Input: part model. Units: mm. Frame: model coordinates. A direction names the side the tool comes from. Coordinates: 2 decimals unless noted, no trailing zeros. Write each loop counter-clockwise with the first axis right and the second up, starting at its lowest first coordinate (ties: lowest second). Pieces come first, ordered by that corner, then holes.
1) Section query C-C (z = -2.25). Output: boundary loops of the cut face in (x, y).
2) Section query B-B (z = 7). Output: boundary loops of the cut face in (x, y).
3) Set-up query: faces 1 (the flat face through (0, 0, 0)), 2 (the cylindrical face through (21.79, 1.05, 5.9)), 3 (the cylindrical face through (-21.79, 0.6, 6.523)). Return all of +Z, -Z, +X, -X, +Y, -Y with unobstructed straight access to the full face (end or side cutting, diameter ignored); none if empty.
4) Draft query along Z for faces 4 (the flat face through (-22.5, 1, 7)), 5 (the cylindrical face through (21.79, 0.6, 6.523)), 6 (the flat face through (0, 1, -8.5)). Return one class per face: pulls with the +Z half, pulls with the -Z half, needs draft (parallel to the pull), parting line crosses it, or undercut.
5) Line query: L1, parallel to X at y = 0.95, z = -5.75; L2, parallel to Z at x = 21.5, y = 0.55. Output: solid intervals per line, ascending.
from build123d import *

# Parameters (mm, degrees)
SKETCH1_W           = 42
SKETCH1_H           = 17
BOSS_EXTRUDE1_DEPTH = 1.5
SKETCH2_R           = 0.5
BOSS_EXTRUDE2_DEPTH = 1.5
FILLET1_R           = 0.1


with BuildPart() as part:
    # Sketch1 → Boss-Extrude1 (new body)
    with BuildSketch(Plane(origin=(0, 0, 0), x_dir=(1, 0, 0), z_dir=(0, 1, 0))):
        Rectangle(SKETCH1_W, SKETCH1_H)
    extrude(amount=BOSS_EXTRUDE1_DEPTH)

    # Sketch2 → Boss-Extrude2 (add)
    with BuildSketch(Plane.ZY.offset(21)):
        with Locations(Location((5.5, 0.75, 0), (0, 0, 180))):
            Circle(SKETCH2_R)
        with Locations(Location((7, 0.75, 0), (0, 0, 180))):
            Circle(SKETCH2_R)
    boss_extrude2 = extrude(amount=BOSS_EXTRUDE2_DEPTH)

    # Mirror1: Boss-Extrude2 across plane
    add(boss_extrude2.mirror(Plane(origin=(0, 0, 0), x_dir=(0, 0, 1), z_dir=(1, 0, 0))))

    # Fillet1
    fillet1_edges = [part.edges().sort_by_distance(p)[0] for p in [
        (21, 1.5, 0),
        (-21, 0.75, 7.5),
        (-21, 0.75, 6),
        (0, 1.5, -8.5),
        (21, 0.75, 6),
        (21, 0.75, 7.5),
        (-21, 1.5, 0),
        (0, 0, -8.5),
        (21, 0, 0),
        (0, 0, 8.5),
        (-21, 0, 0),
        (-21, 0.75, -8.5),
        (21, 0.75, -8.5),
        (21, 0.75, 8.5),
        (-21, 0.75, 8.5),
        (0, 1.5, 8.5),
    ]]
    fillet(fillet1_edges, radius=FILLET1_R)


solid = part.part
Answer:
1. outline: (-21, 0.1) arc R0.1 ccw to (-20.9, 0) - (20.9, 0) arc R0.1 ccw to (21, 0.1) - (21, 1.4) arc R0.1 ccw to (20.9, 1.5) - (-20.9, 1.5) arc R0.1 ccw to (-21, 1.4) - close
2. outline: (-22.5, 0.25) - (-21.1, 0.25) arc R0.1 cw to (-21, 0.15) - (-21, 0.1) arc R0.1 ccw to (-20.9, 0) - (20.9, 0) arc R0.1 ccw to (21, 0.1) - (21, 0.15) arc R0.1 cw to (21.1, 0.25) - (22.5, 0.25) - (22.5, 1.25) - (21.1, 1.25) arc R0.1 cw to (21, 1.35) - (21, 1.4) arc R0.1 ccw to (20.9, 1.5) - (-20.9, 1.5) arc R0.1 ccw to (-21, 1.4) - (-21, 1.35) arc R0.1 cw to (-21.1, 1.25) - (-22.5, 1.25) - close
3. face 1: +Z, -Z, +X, -X, -Y
3. face 2: +X
3. face 3: -X
4. face 4: needs draft
4. face 5: undercut
4. face 6: pulls with the -Z half
5. L1: x = -21 to 21
5. L2: z = 5.04 to 5.96, 6.54 to 7.46
